Geometry: see drawing. Coordinates: mm, zero at the bounding-box minimum. A direction names the side the tool comes from. Give positions to 0.01 mm unless a question says otherwise; leave off trailing zeros. Write each loop counter-clockwise with the first axis right and the second up, starting at its lowest first coordinate (ties: lowest second). Pieces come first, ordered by that corner, then holes. Notation, with made-up numbers: M 50.25,88.25 L 83.25,88.25 A27 cw 83.25,122.25 Z; hole C 10.25,26.5 d11. An arc over 180 degrees is marked long. Use a Markdown table: item, result. Add a question column.
1) Section B-B on x = 76.2. Return the cut outline in (y, z).
2) Section D-D on x = 138. Return the cut outline in (y, z) (1 decimal), then the cut area to 3 significant figures.
3) Section A-A on z = 76.2. Return the cut outline in (x, y), then the cut area to 3 significant figures.
4) Section C-C on y = 44.5. Return the cut outline in (x, z).
5) Set-up query: the marked faces 1, 2, 3, 4 and 5. Return all of +Z, -Z, +X, -X, +Y, -Y with unobstructed straight access to the full face (end or side cutting, diameter ignored); none if empty.
6) Pin query (flat end, axial travel): pin 1 (4 mm diameter, centred on y = 85, z = 99.5, fed in from +X) (1 decimal); pin 2 (6 mm diameter, centred on x = 98, y = 10, fed in from +Z); pin 3 (12 mm diameter, centred on x = 74, z = 110.5, fed in from -Y); pin 4 (12 mm diameter, centred on x = 119.5, y = 33, fed in from -Z). Return the tip coordinate at first contact, or that it passes through.
7) Draft query along X for the marked faces 6, 7, 8 and 9. Return one class per face: +X half, -X half, draft (parallel to the pull), parting line (faces both ways), or undercut.
8) Line query: line 1 (X direction, y = 25, z = 32) (1 decimal); line 2 (X direction, y = 49, z = 47.5) (1 decimal); line 3 (Z direction, x = 81, y = 61.5). Output: solid intervals per line, ascending.
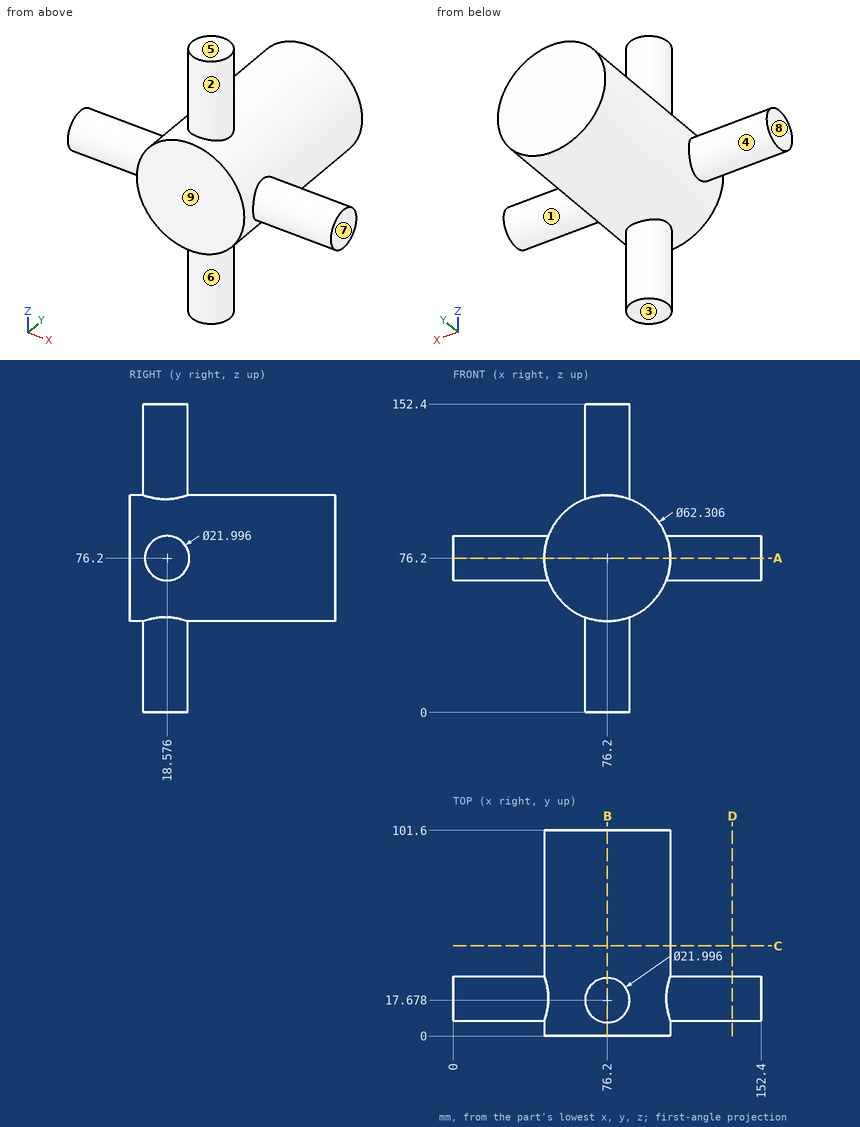
Found:
| question | item | result |
|---|---|---|
| 1 | outline | M 0,45.05 L 6.68,45.05 L 6.68,0 L 28.68,0 L 28.68,45.05 L 101.6,45.05 L 101.6,107.35 L 28.68,107.35 L 28.68,152.4 L 6.68,152.4 L 6.68,107.35 L 0,107.35 Z |
| 2 | outline | C 18.6,76.2 d22 |
| 2 | area | 380 mm² |
| 3 | outline | M 0,7.58 L 45.05,7.58 L 45.05,0 L 107.35,0 L 107.35,7.58 L 152.4,7.58 L 152.4,29.57 L 107.35,29.57 L 107.35,101.6 L 45.05,101.6 L 45.05,29.57 L 0,29.57 Z |
| 3 | area | 8,310 mm² |
| 4 | outline | C 76.2,76.2 d62.31 |
| 5 | face 1 | +X |
| 5 | face 2 | +Z |
| 5 | face 3 | -Z, +X, -X, +Y, -Y |
| 5 | face 4 | -X |
| 5 | face 5 | +Z, +X, -X, +Y, -Y |
| 6 | pin 1 | x = 98.9 |
| 6 | pin 2 | z = 101.04 |
| 6 | pin 3 | y = 0 |
| 6 | pin 4 | z = 69.13 |
| 7 | face 6 | parting line |
| 7 | face 7 | +X half |
| 7 | face 8 | -X half |
| 7 | face 9 | draft |
| 8 | line 1 | 68 to 84.4 |
| 8 | line 2 | 64.1 to 88.3 |
| 8 | line 3 | 45.42 to 106.98 |
